```python
from build123d import *

# Parameters (mm, degrees)
BOSS_EXTRUDE1_DEPTH = 50
SKETCH2_R           = 9.5
CUT_EXTRUDE1_DEPTH  = 10
M3_TAPPED_HOLE1_D   = 2.5
SKETCH7_R           = 2.15
CUT_EXTRUDE2_DEPTH  = 10
FILLET1_R           = 3
FILLET2_R           = 6
FILLET3_R           = 15
FILLET4_R           = 8


with BuildPart() as part:
    # Sketch1 → Boss-Extrude1 (new body)
    with BuildSketch(Plane.XY):
        Polygon((-54, 0), (-30, 0), (-30, 20), (30, 20), (30, 0), (54, 0), (54, 4), (34, 4), (34, 24), (-34, 24), (-34, 4), (-54, 4), align=None)
    extrude(amount=BOSS_EXTRUDE1_DEPTH)

    # Sketch2 → Cut-Extrude1 (cut)
    with BuildSketch(Plane(origin=(0, 24, 0), x_dir=(1, 0, 0), z_dir=(0, 1, 0))):
        with Locations(Location((0, -25, 0), (0, 0, 270))):
            Circle(SKETCH2_R)
    extrude(amount=-CUT_EXTRUDE1_DEPTH, mode=Mode.SUBTRACT)

    # M3 Tapped Hole1 (through all)
    with Locations(Plane(origin=(0, 24, 0), x_dir=(1, 0, 0), z_dir=(0, 1, 0))):
        with Locations((20, -25), (-20, -25)):
            Hole(M3_TAPPED_HOLE1_D / 2)

    # Sketch7 → Cut-Extrude2 (cut)
    with BuildSketch(Plane(origin=(0, 4, 0), x_dir=(1, 0, 0), z_dir=(0, 1, 0))):
        with Locations(Location((-44, -44, 0), (0, 0, 180))):
            Circle(SKETCH7_R)
        with BuildLine():
            ThreePointArc((46.25, -44), (45.906571503, -36.134194217), (44.878899709, -28.328251966))
            ThreePointArc((44.878899709, -28.328251966), (42.272373865, -26.503142921), (40.447264821, -29.109668765))
            ThreePointArc((40.447264821, -29.109668765), (41.423695361, -36.526395059), (41.75, -44))
            ThreePointArc((41.75, -44), (44, -46.25), (46.25, -44))
        make_face()
        with BuildLine():
            ThreePointArc((48.004434954, -19.347485954), (45.50572213, -11.422581348), (42.325816715, -3.745610569))
            ThreePointArc((42.325816715, -3.745610569), (39.335733105, -2.657309137), (38.247431674, -5.647392747))
            ThreePointArc((38.247431674, -5.647392747), (41.277105336, -12.961671993), (43.657768736, -20.512171657))
            ThreePointArc((43.657768736, -20.512171657), (46.413444696, -22.103161915), (48.004434954, -19.347485954))
        make_face()
    extrude(amount=-CUT_EXTRUDE2_DEPTH, mode=Mode.SUBTRACT)

    # Fillet1
    fillet1_edges = [part.edges().sort_by_distance(p)[0] for p in [
        (-34, 4, 25),
        (34, 4, 25),
        (30, 20, 25),
        (-30, 20, 25),
    ]]
    fillet(fillet1_edges, radius=FILLET1_R)

    # Fillet2
    fillet2_edges = [part.edges().sort_by_distance(p)[0] for p in [
        (-34, 24, 25),
        (34, 24, 25),
        (30, 0, 25),
        (-30, 0, 25),
    ]]
    fillet(fillet2_edges, radius=FILLET2_R)

    # Fillet3
    fillet3_edges = [part.edges().sort_by_distance(p)[0] for p in [
        (-54, 2, 0),
    ]]
    fillet(fillet3_edges, radius=FILLET3_R)

    # Fillet4
    fillet4_edges = [part.edges().sort_by_distance(p)[0] for p in [
        (54, 2, 0),
        (54, 2, 50),
        (-54, 2, 50),
    ]]
    fillet(fillet4_edges, radius=FILLET4_R)


solid = part.part
```
For this review, take the finished solid that the model builds, in its own axes (mm). A direction names the side the tool comes from. Round coordinates to 2 decimals unless told otherwise and drop trailing zeros. Loops run counter-clockwise (first coordinate to the right, second up) from the corner with the lowest first, then second, coordinate; pieces in that order, holes last.
(1) We need section C-C (x = -20). Give the boundary of the cut face in (y, z).
Returned:
outline: (20, 0) - (24, 0) - (24, 23.75) - (20, 23.75) - close; (20, 26.25) - (24, 26.25) - (24, 50) - (20, 50) - close
(2) We need section A-A (y = 14.5). Give the boundary of the cut face in (x, z), plus the area to 3 significant figures.
Returned:
outline: (-34, 0) - (-30, 0) - (-30, 50) - (-34, 50) - close; (30, 0) - (34, 0) - (34, 50) - (30, 50) - close
area: 400 mm2
(3) We need section B-B (z = 25). State how many separate pieces and enclosed holes the cut face has, plus the area to 3 significant figures.
Returned:
separate pieces: 4
enclosed holes: 0
area: 473 mm2
(4) Mouldability with a two-part tool opening along Z and no side actions: class faces 1 (the cylindrical face through (42.3, 2, 26.5)), 2 (the cylindrical face through (-51.719, 1.972, 47.594)), 3 (the flat face through (45, 0, 25)), 4 (the cylindrical face through (45.916, 2.028, 36.244)) as released by +Z, released by -Z, zero draft, split by the parting line, or undercut.
Returned:
face 1: undercut
face 2: released by +Z
face 3: zero draft
face 4: undercut
(5) Tool access review of faces 5 (the flat face through (-45, 4, 25)), 6 (the flat face through (-45, 0, 25)), 7 (the cylindrical face through (45.545, 2.028, 11.532)), 8 (the cylindrical face through (29.1, 19.14, 25.35)): name each direction out of +Z, -Z, +X, -X, +Y, -Y from which nothing blocks a thin tool from reaching the whole face with its end or side.
Returned:
face 5: +Z, -Z, -X, +Y
face 6: +Z, -Z, +X, -X, -Y
face 7: +Y, -Y
face 8: +Z, -Z, -Y
(6) We need section D-D (y = 2). Give the boundary of the cut face in (x, z), plus the area to 3 significant figures.
Returned:
outline: (-54, 15) arc R15 ccw to (-39, 0) - (-31.53, 0) - (-31.53, 50) - (-46, 50) arc R8 ccw to (-54, 42) - close; (31.53, 0) - (46, 0) arc R8 ccw to (54, 8) - (54, 42) arc R8 ccw to (46, 50) - (31.53, 50) - close; hole circle Ø4.3 at (-44, 44); hole (38.25, 5.65) arc R2.25 ccw to (42.33, 3.75) arc R95.25 ccw to (48, 19.35) arc R2.25 ccw to (43.66, 20.51) arc R90.75 cw to start; hole (40.45, 29.11) arc R2.25 ccw to (44.88, 28.33) arc R90.25 ccw to (46.25, 44) arc R2.25 ccw to (41.75, 44) arc R85.75 cw to start
area: 1,970 mm2
(7) Clearance check with flat-ended pins moving along their axes: P1, Ø5, axis at x = -49, z = 28.5, coming from the +Y side; P2, Ø3.5, axis at x = -44, z = 44, coming from the +Y side; P3, Ø9, axis at y = 12, z = 30.5, coming from the -X side; P4, Ø13.5, axis at x = 41.5, z = 18, coming from the +Y side. State where each tip first meets the part, or that it passes through.
Returned:
P1: stops at y = 4
P2: passes through
P3: stops at x = -34
P4: stops at y = 5.02
(8) Wall thickness on line 1 along X through (y, z) = (14.5, 39); line 2 along X through (y, z) = (23, 25); line 3 along Z through (x, y) = (20, 22.65): over which ranges is each line inside the solid? List them lowest first.
Returned:
line 1: x = -34 to -30, 30 to 34
line 2: x = -31.32 to -21.25, -18.75 to -9.5, 9.5 to 18.75, 21.25 to 31.32
line 3: z = 0 to 23.75, 26.25 to 50
